```python
from build123d import *

# Parameters (mm, degrees)
F0_W     = 44
F0_H     = 115
F1_DEPTH = 5
F5_W     = 2
F5_H     = 7.4
F6_DEPTH = 44.001
F7_W     = 44
F7_H     = 8.75
F7_H_2   = 21.35
F8_DEPTH = 2


with BuildPart() as f1:
    # F0 (on Front) → F1 (new body)
    with BuildSketch(Plane.XZ):
        Rectangle(F0_W, F0_H)
    extrude(amount=F1_DEPTH)

    # F5 (on face) → F6 (cut, through all)
    with BuildSketch(Plane.YZ.offset(22)):
        with Locations((-4, 53.8)):
            Rectangle(F5_W, F5_H)
    extrude(amount=-F6_DEPTH, mode=Mode.SUBTRACT)

    # F7 (on face) → F8 (cut)
    with BuildSketch(Plane.XZ.offset(5)):
        with Locations((0, 35.475)):
            Rectangle(F7_W, F7_H)
        with Locations((0, 16.475)):
            Rectangle(F7_W, F7_H)
        with Locations((0, -2.525)):
            Rectangle(F7_W, F7_H)
        with Locations((0, -21.525)):
            Rectangle(F7_W, F7_H)
        with Locations((0, -46.825)):
            Rectangle(F7_W, F7_H_2)
    extrude(amount=-F8_DEPTH, mode=Mode.SUBTRACT)


solid = f1.part
```
Input: part model. Units: mm. Frame: model coordinates. A direction names the side the tool comes from. Give positions to 0.01 mm unless a question says otherwise; leave off trailing zeros. Order: outer loops, then holes, each group sorted by start corner. A loop starts at its lowest first (then second) coordinate and runs counter-clockwise, first axis right, second up.
1. Set-up query: faces 4 (the face through (0, -3, 36)), 5 (the face through (0, -5, 7)), 6 (the face through (0, -4, -36.15)). Return all of +Z, -Z, +X, -X, +Y, -Y with unobstructed straight access to the full face (end or side cutting, diameter ignored); none if empty.
Computed:
face 4: +X, -X, -Y
face 5: +Z, -Z, +X, -X, -Y
face 6: -Z, +X, -X, -Y
2. Cut plane B-B (x = 19). Return loops of the section in (y, z), and give its area (4 significant figures).
Computed:
outline: (-5, -36.15) - (-3, -36.15) - (-3, -57.5) - (0, -57.5) - (0, 57.5) - (-3, 57.5) - (-3, 50.1) - (-5, 50.1) - (-5, 39.85) - (-3, 39.85) - (-3, 31.1) - (-5, 31.1) - (-5, 20.85) - (-3, 20.85) - (-3, 12.1) - (-5, 12.1) - (-5, 1.85) - (-3, 1.85) - (-3, -6.9) - (-5, -6.9) - (-5, -17.15) - (-3, -17.15) - (-3, -25.9) - (-5, -25.9) - close
area: 447.5 mm2
3. Pin query (flat end, axial travel): pin 1 Ø0.6 at (x, y) = (8.5, -4) entering from +Z; pin 2 Ø1.6 at (x, y) = (8.5, -4.5) entering from -Z; pin 3 Ø5 at (x, z) = (-4, -2) entering from -Y. Return the tip coordinate at first contact, or that it passes through.
Computed:
pin 1: stops at z = 50.1
pin 2: stops at z = -36.15
pin 3: stops at y = -3
4. Line query: probe 1 along Z at (x, y) = (-17.5, -4.05); probe 2 along Y at (x, z) = (-20, 0.5). Output: solid intervals per line, ascending.
Computed:
probe 1: z = -36.15 to -25.9, -17.15 to -6.9, 1.85 to 12.1, 20.85 to 31.1, 39.85 to 50.1
probe 2: y = -3 to 0
5. Draft query along Z for faces 1 (the face through (-22, -2, -1)), 2 (the face through (0, -4, 31.1)), 3 (the face through (0, -1, 57.5)). Return one class per face: released by +Z, released by -Z, zero draft, split by the parting line, or undercut.
Computed:
face 1: zero draft
face 2: undercut
face 3: released by +Z
6. Cut plane A-A (y = -4.05). Return loops of the section in (x, z), and give its area (4 significant figures).
Computed:
outline: (-22, -36.15) - (22, -36.15) - (22, -25.9) - (-22, -25.9) - close; (-22, -17.15) - (22, -17.15) - (22, -6.9) - (-22, -6.9) - close; (-22, 1.85) - (22, 1.85) - (22, 12.1) - (-22, 12.1) - close; (-22, 20.85) - (22, 20.85) - (22, 31.1) - (-22, 31.1) - close; (-22, 39.85) - (22, 39.85) - (22, 50.1) - (-22, 50.1) - close
area: 2,255 mm2
7. Cut plane C-C (z = -21.5). Return loops of the section in (x, y), and give its area (3 significant figures).
Computed:
outline: (-22, -3) - (22, -3) - (22, 0) - (-22, 0) - close
area: 132 mm2
